```python
from build123d import *

# Parameters (mm, degrees)
F1_DEPTH = 6.35
F3_DEPTH = 25
F4_R     = 5


with BuildPart() as f1:
    # F0 (on Front) → F1 (new body)
    with BuildSketch(Plane.XZ):
        with BuildLine():
            Line((0, -12), (0, -3.2))
            ThreePointArc((0, -3.2), (-2.262742, -2.262742), (-3.2, 0))
            Line((-3.2, 0), (-12, 0))
            Line((-12, 0), (-12, -12))
            Line((-12, -12), (0, -12))
        make_face()
        with BuildLine():
            ThreePointArc((0, 3.2), (2.262742, 2.262742), (3.2, 0))
            ThreePointArc((3.2, 0), (2.262742, -2.262742), (0, -3.2))
            Line((0, -3.2), (0, -12))
            Line((0, -12), (12, -12))
            Line((12, -12), (12, 200))
            Line((12, 200), (0, 200))
            Line((0, 200), (0, 3.2))
        make_face()
        with BuildLine():
            ThreePointArc((-3.2, 0), (-2.262742, 2.262742), (0, 3.2))
            Line((0, 3.2), (0, 200))
            Line((0, 200), (-12, 200))
            Line((-12, 200), (-12, 0))
            Line((-12, 0), (-3.2, 0))
        make_face()
    extrude(amount=F1_DEPTH)

    # F2 (on face) → F3 (cut)
    with BuildSketch(Plane.XZ.offset(6.35)):
        with BuildLine():
            ThreePointArc((0, 193.1), (-2.192031, 187.807969), (3.1, 190))
            ThreePointArc((3.1, 190), (2.192031, 192.192031), (0, 193.1))
        make_face()
    extrude(amount=-F3_DEPTH, mode=Mode.SUBTRACT)

    # F4
    f4_edges = [f1.edges().sort_by_distance(p)[0] for p in [
        (12, -3.175, 200),
        (-12, -3.175, 200),
        (12, -3.175, -12),
        (-12, -3.175, -12),
    ]]
    fillet(f4_edges, radius=F4_R)


solid = f1.part
```
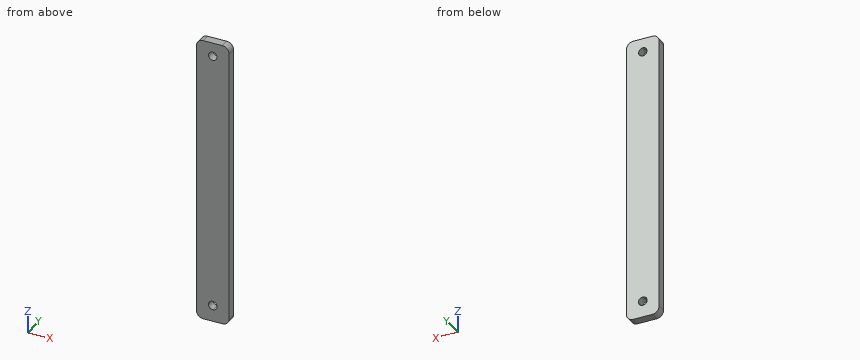
Model file for the job. Use its own axes, mm. Round coordinates to 2 decimals unless told otherwise and drop trailing zeros. Write each loop counter-clockwise with the first axis right and the second up, starting at its lowest first coordinate (ties: lowest second). Pieces come first, ordered by that corner, then holes. Notation, with made-up numbers: (18, 44) - (69, 44) arc R7 ccw to (69, 55) - close; hole circle Ø7 at (52, 25). An arc over 180 degrees is marked (long way). Use CSV: the item, a comma, the result in double quotes. Start each with the question number.
Item 1: Band-saw the part on A-A (y = -5). Write the cut outline in (x, z), and give its area (3 significant figures).
Item 2: Pin check, flat tip, straight feed: P1, Ø3, axis at x = -9, y = -5.5, coming from the -Z side. Stop position of the tip, or through.
Item 3: Drill centre lines: L1, parallel to Z at x = 0, y = -1.75; L2, parallel to Z at x = 1, y = -3; L3, parallel to X at y = -4, z = 190. Where is each one in solid material? Low to high. Write a range as [from, to].
Checked values:
1,outline,"(-12, -7) arc R5 ccw to (-7, -12) - (7, -12) arc R5 ccw to (12, -7) - (12, 195) arc R5 ccw to (7, 200) - (-7, 200) arc R5 ccw to (-12, 195) - close; hole (-3.2, 0) arc R3.2 ccw to (0, -3.2) arc R3.2 ccw to (3.2, 0) arc R3.2 ccw to (0, 3.2) arc R3.2 ccw to start; hole circle Ø6.2 at (0, 190)"
1,area,"5,000 mm²"
2,P1,"stops at z = -11.97"
3,L1,"z = [-12, -3.2], [3.2, 186.9], [193.1, 200]"
3,L2,"z = [-12, -3.04], [3.04, 187.07], [192.93, 200]"
3,L3,"x = [-12, -3.1], [3.1, 12]"
